Could you check a few things on this model? Use its own coordinates, in mm. Face numbers are marked on the shaded views. Give positions to 0.01 mm unless a question says otherwise; leave off trailing zeros. Loops run counter-clockwise (first coordinate to the right, second up) from the corner with the lowest first, then second, coordinate; pieces in that order, holes last. Notation, with made-up numbers: M 50.25,19.25 L 88.25,19.25 A31 ccw 88.25,55.25 Z; hole C 62,-34 d7. An arc over 180 degrees is marked long. Return JSON: item names as keys, results as strings. Group by question number.
1. If we mould it in two halves opening along Z, with no side actions, what happens to the marked faces 1 and 2? For each: +Z half, -Z half, draft (parallel to the pull), parting line (faces both ways), or undercut.
2. If we section it at B-B (y = 121.5): State how many separate pieces and enclosed holes the cut face has, plus the area to 3 significant figures.
3. If we section it at A-A (x = 0): Write out the boundary of the cut face in (y, z), plus the area to 3 significant figures.
4. For pin 1 (2.5 mm diameter, centred on x = 8.5, z = 120.5, fed in from +Y); pin 2 (1 mm diameter, centred on x = 35, y = 105.5, fed in from -Z); pin 3 (7 mm diameter, centred on x = 14.5, z = 126.5, fed in from -Y); pin 4 (10 mm diameter, centred on x = 27, y = 84, fed in from -Z), each with a flat end and sliding along its axis, tell me the tip position at first contact or that it passes through.
5. If we section it at C-C (z = 0): Write out the boundary of the cut face in (x, y).
6. Please list where these lines run through material, in increasing order: line 1 (X direction, y = 142.5, z = 81); line 2 (Z direction, x = -110, y = 10.5); line 3 (X direction, y = 132.5, z = -20.5).
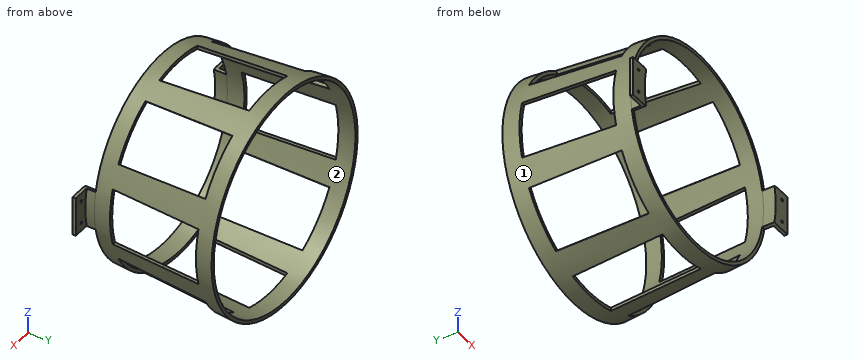
```python
from build123d import *

# Parameters (mm, degrees)
SKETCH6_W           = 70
SKETCH6_H           = 110
CUT_EXTRUDE2_DEPTH  = 20
BOSS_EXTRUDE1_DEPTH = 15
BOSS_EXTRUDE2_DEPTH = 4
SKETCH9_R           = 1.6
CUT_EXTRUDE3_DEPTH  = 24
CIRPATTERN1_COUNT   = 8


with BuildPart() as part:
    # Sketch2 → Revolve1 (revolve)
    with BuildSketch(Plane.XY):
        Polygon((120, 0), (130, 150), (134.008879034, 150), (124.008879034, 0), align=None)
    revolve(axis=Axis((0, 0, 0), (0, 1, 0)))

    # Sketch6 → Cut-Extrude2 (cut, symmetric)
    with BuildSketch(Plane.XY.offset(134)):
        with Locations((0, 75)):
            Rectangle(SKETCH6_W, SKETCH6_H)
    cut_extrude2 = extrude(amount=CUT_EXTRUDE2_DEPTH, both=True, mode=Mode.SUBTRACT)

    # Sketch7 → Boss-Extrude1 (add)
    with BuildSketch(Plane(origin=(0, 0, 0), x_dir=(1, 0, 0), z_dir=(0, 1, 0))):
        with BuildLine():
            Line((-117.744298431, 23.157724131), (-121.677820509, 23.931361754))
            ThreePointArc((-121.677820509, 23.931361754), (-124.008879034, 0), (-121.677820509, -23.931361754))
            Line((-121.677820509, -23.931361754), (-117.744298431, -23.157724131))
            ThreePointArc((-117.744298431, -23.157724131), (-120, 0), (-117.744298431, 23.157724131))
        make_face()
        with BuildLine():
            Line((117.744298431, -23.157724131), (121.677820509, -23.931361754))
            ThreePointArc((121.677820509, -23.931361754), (124.008879034, 0), (121.677820509, 23.931361754))
            Line((121.677820509, 23.931361754), (117.744298431, 23.157724131))
            ThreePointArc((117.744298431, 23.157724131), (120, 0), (117.744298431, -23.157724131))
        make_face()
    extrude(amount=-BOSS_EXTRUDE1_DEPTH)

    # Sketch8 → Boss-Extrude2 (add)
    with BuildSketch(Plane.XZ.offset(15)):
        with BuildLine():
            Line((121.677820509, 23.931361754), (141.677820509, 23.931361754))
            Line((141.677820509, 23.931361754), (141.677820509, -23.931361754))
            Line((141.677820509, -23.931361754), (121.677820509, -23.931361754))
            ThreePointArc((121.677820509, -23.931361754), (124.008879034, 0), (121.677820509, 23.931361754))
        make_face()
        with BuildLine():
            Line((-121.677820509, 23.931361754), (-141.677820509, 23.931361754))
            Line((-141.677820509, 23.931361754), (-141.677820509, -23.931361754))
            Line((-141.677820509, -23.931361754), (-121.677820509, -23.931361754))
            ThreePointArc((-121.677820509, -23.931361754), (-124.008879034, 0), (-121.677820509, 23.931361754))
        make_face()
    extrude(amount=-BOSS_EXTRUDE2_DEPTH)

    # Sketch9 → Cut-Extrude3 (cut)
    with BuildSketch(Plane.XZ.offset(15)):
        with Locations((131.677820509, 13.931361754)):
            Circle(SKETCH9_R)
        with Locations((131.677820509, -13.931361754)):
            Circle(SKETCH9_R)
        with Locations((-131.677820509, -13.931361754)):
            Circle(SKETCH9_R)
        with Locations((-131.677820509, 13.931361754)):
            Circle(SKETCH9_R)
    extrude(amount=-CUT_EXTRUDE3_DEPTH, mode=Mode.SUBTRACT)

    # CirPattern1: Cut-Extrude2 ×8 about axis
    cirpattern1_axis = Axis((0, 0, 0), (0, 1, 0))
    for i in range(1, CIRPATTERN1_COUNT):
        add(cut_extrude2.rotate(cirpattern1_axis, i * 360 / CIRPATTERN1_COUNT), mode=Mode.SUBTRACT)


solid = part.part
```
Answer:
{
 "1": {"face 1": "parting line", "face 2": "undercut"},
 "2": {"separate pieces": "8", "enclosed holes": "0", "area": "1,000 mm²"},
 "3": {"outline": "M 0,-124.01 L 20,-125.34 L 20,-121.33 L 0,-120 Z; M 0,120 L 20,121.33 L 20,125.34 L 0,124.01 Z; M 130,-132.68 L 150,-134.01 L 150,-130 L 130,-128.67 Z; M 130,128.67 L 150,130 L 150,134.01 L 130,132.68 Z", "area": "321 mm²"},
 "4": {"pin 1": "stops at y = 20", "pin 2": "stops at z = -126.32", "pin 3": "stops at y = 0", "pin 4": "passes through"},
 "5": {"outline": "M -141.68,-15 L -120,-15 L -120,0 L -121.33,20 L -125.34,20 L -124.01,0 L -124.01,-11 L -141.68,-11 Z; M -134.01,150 L -132.68,130 L -128.67,130 L -130,150 Z; M 120,-15 L 141.68,-15 L 141.68,-11 L 124.01,-11 L 124.01,0 L 125.34,20 L 121.33,20 L 120,0 Z; M 128.67,130 L 132.68,130 L 134.01,150 L 130,150 Z"},
 "6": {"line 1": "x = -106.13 to -101.04, 101.04 to 106.13", "line 2": "z = -58.76 to -49.68, 49.68 to 58.76", "line 3": "x = -131.25 to -127.19, 127.19 to 131.25"}
}
